Autodesk Inventor part; units mm, degrees
ref_plane "YZ Plane" through (0, 0, 0) normal (1, 0, 0) x (0, 1, 0)
ref_plane "XZ Plane" through (0, 0, 0) normal (0, 1, 0) x (-1, 0, 0)
ref_plane "XY Plane" through (0, 0, 0) normal (0, 0, 1) x (1, 0, 0)
sketch "Sketch1" plane through (0, 0, 0) normal (0, 0, 1) x (1, 0, 0)
  line L0 (-15, -10) -> (15, -10)
  line L1 (15, -10) -> (15, 10)
  line L2 (15, 10) -> (-15, 10)
  line L3 (-15, 10) -> (-15, -10)
  line L4 (-15, -10) -> (15, 10) construction
  line L5 (15, -10) -> (-15, 10) construction
  point P0 (0, 0)
  dimension "d0" = 30
  dimension "d1" = 20
extrude "Extrusion1" add sketch "Sketch1" against normal blind 5
sketch "Sketch2" plane through (0, 0, 0) normal (0, 0, 1) x (1, 0, 0)
  line L0 (-15, 0) -> (15, 0)
  line L1 (15, 0) -> (15, 15)
  line L2 (15, 15) -> (-15, 15)
  line L3 (-15, 15) -> (-15, 0)
  line L4 (-15, 0) -> (15, 15) construction
  line L5 (15, 0) -> (-15, 15) construction
  line L6 (15, 10) -> (-15, 10)
  line L7 (-15, 10) -> (-15, -10)
  point P0 (0, 0)
  point P1 (0, 7.5)
  dimension "d4" = 30
  dimension "d5" = 15
  dimension "d18" = 5
extrude "Extrusion2" add sketch "Sketch2" along normal blind 15
sketch "Sketch3" plane through (0, 0, 0) normal (0, 0, 1) x (1, 0, 0)
  circle A0 centre (10, -10) radius 2
  circle A1 centre (-10, -10) radius 2
  line L0 (-15, -10) -> (15, -10)
  line L1 (-15, 0) -> (-15, -10)
  point P0 (0, 0)
  dimension "d8" = 4
  dimension "d9" = 4
  dimension "d12" = 5
  dimension "d13" = 20
sketch "Sketch4" plane through (-15, -10, 0) normal (0, -1, 0) x (1, 0, 0)
  line L0 (0, -5) -> (30, -5)
  line L1 (30, -5) -> (30, 0)
  line L2 (30, 0) -> (0, 0)
  line L3 (0, 0) -> (0, -5)
  line L4 (0, -5) -> (30, 0) construction
  line L5 (30, -5) -> (0, 0) construction
  line L6 (0, 0) -> (30, 0)
  line L7 (30, 0) -> (30, -5)
  line L8 (0, 0) -> (0, -5)
  line L9 (30, -5) -> (0, -5)
  point P0 (15, 0)
  point P1 (15, -2.5)
extrude "Extrusion3" add sketch "Sketch4" along normal blind 5
extrude "Extrusion4" cut sketch "Sketch3" against normal blind 5
sketch "Sketch5" plane through (0, 0, -5) normal (0, 0, -1) x (-1, 0, 0)
  line L0 (-8, 0) -> (8, 0)
  line L1 (8, 0) -> (8, 15)
  line L2 (8, 15) -> (-8, 15)
  line L3 (-8, 15) -> (-8, 0)
  line L4 (-8, 0) -> (8, 15) construction
  line L5 (8, 0) -> (-8, 15) construction
  line L6 (-15, 15) -> (15, 15)
  point P0 (0, 0)
  point P1 (0, 7.5)
  dimension "d16" = 16
  dimension "d21" = 15
  dimension "d22" = 0
sketch "Sketch6" plane through (0, 0, 0) normal (0, 0, -1) x (-1, 0, 0)
  line L0 (-15, 10) -> (15, 10)
  line L1 (15, 10) -> (15, 15)
  line L2 (15, 15) -> (-15, 15)
  line L3 (-15, 15) -> (-15, 10)
  line L4 (-15, 10) -> (15, 15) construction
  line L5 (15, 10) -> (-15, 15) construction
  line L6 (-15, 15) -> (15, 15)
  line L7 (15, 10) -> (-15, 10)
  line L8 (-15, 10) -> (-15, 15)
  line L9 (15, 15) -> (15, 10)
  point P0 (0, 0)
  point P1 (0, 12.5)
extrude "Extrusion5" add sketch "Sketch6" along normal blind 5
extrude "Extrusion6" cut sketch "Sketch5" against normal through all
sketch "Sketch7" plane through (0, 0, -5) normal (0, 0, -1) x (-1, 0, 0)
  circle A0 centre (-10, 8) radius 1.5
  circle A1 centre (10, 8) radius 1.5
  line L0 (-15, 15) -> (-15, -15)
  line L1 (8, 0) -> (-8, 0)
  point P0 (0, 0)
  dimension "d25" = 3
  dimension "d26" = 3
  dimension "d27" = 20
  dimension "d28" = 5
  dimension "d33" = 8
extrude "Extrusion7" cut sketch "Sketch7" against normal through all
sketch "Sketch8" plane through (15, 15, 15) normal (0, 1, 0) x (1, 0, 0)
  line L0 (0, 20) -> (-30, 20)
  line L1 (-30, 20) -> (-30, 0)
  line L2 (-30, 0) -> (0, 0)
  line L3 (0, 0) -> (0, 20)
  line L4 (0, 20) -> (-30, 0) construction
  line L5 (-30, 20) -> (0, 0) construction
  line L6 (0, 0) -> (-7, 0)
  line L7 (0, 0) -> (0, 20)
  line L8 (-23, 20) -> (-7, 20)
  line L9 (-30, 20) -> (-30, 0)
  point P0 (-15, 15)
  point P1 (-15, 10)
extrude "Extrusion8" add sketch "Sketch8" along normal blind 3
sketch "Sketch9" plane through (0, 0, -5) normal (0, 0, -1) x (-1, 0, 0)
  line L0 (-13, 4) -> (-8, 4)
  line L1 (-8, 4) -> (-8, 12)
  line L2 (-8, 12) -> (-13, 12)
  line L3 (-13, 12) -> (-13, 4)
  line L4 (-13, 4) -> (-8, 12) construction
  line L5 (-8, 4) -> (-13, 12) construction
  line L6 (8, 4) -> (13, 4)
  line L7 (13, 4) -> (13, 12)
  line L8 (13, 12) -> (8, 12)
  line L9 (8, 12) -> (8, 4)
  line L10 (8, 4) -> (13, 12) construction
  line L11 (13, 4) -> (8, 12) construction
  line L12 (-8, 0) -> (-8, 15)
  line L13 (8, 15) -> (8, 0)
  line L14 (8, 0) -> (-8, 0)
  point P0 (0, 0)
  point P1 (-10.5, 8)
  point P2 (10.5, 8)
  dimension "d34" = 5
  dimension "d35" = 5
  dimension "d36" = 8
  dimension "d37" = 8
  dimension "d38" = 8
extrude "Extrusion9" cut sketch "Sketch9" against normal blind 10
fillet "Fillet1" radius 3 2 edges at (15, 18, 5) (-15, 18, 5)
fillet "Fillet2" radius 3 3 edges at (15, 7.5, 15) (-15, 7.5, 15) (0, 18, 15)
properties part number "IR_bracket"
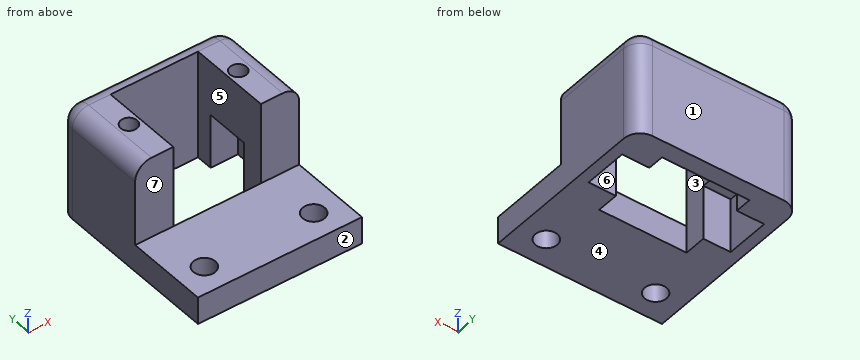
Model file for the job. Use its own axes, mm. Face numbers are marked on the shaded views. A direction names the side the tool comes from. Coordinates: 2 decimals unless noted, no trailing zeros. Write each loop counter-clockwise with the first axis right and the second up, starting at its lowest first coordinate (ties: lowest second). Pieces come first, ordered by that corner, then holes. Notation, with made-up numbers: (46.25, 52.25) - (50.25, 52.25) arc R12 cw to (50.25, 75.25) - close; hole circle Ø1 at (51.25, 54.25). An arc over 180 degrees is marked (long way). One line per item, written item: value. Start each with the question number.
1. Flat gauge pins, fed straight in: pin 1 (1.5 mm diameter, centred on x = 11, y = 7.5, fed in from -Z); pin 2 (2 mm diameter, centred on x = -12, z = 7.5, fed in from -Y); pin 3 (4.5 mm diameter, centred on x = 3.5, y = -4.5, fed in from +Z). Where does each tip first touch, or does it go through?
2. Slice it at A-A (x = 10). Write the cut outline in (y, z), plus the area to 3 significant figures.
3. Tool access for the marked faces 5, 6 and 7: list every direction of +Z, -Z, +X, -X, +Y, -Y with a clear straight run to the whole face (end or side of a thin tool).
4. Slice it at D-D (z = 11.5). Write the cut outline in (x, y), plus the area to 3 significant figures.
5. Slice it at B-B (y = 8). Write the cut outline in (x, z), plus the area to 3 significant figures.
6. Probe line 1 (Y direction, x = 10, z = -1.2); line 2 (X direction, y = -10, z = -3.9); line 3 (X direction, y = 4, z = 6.5). List the from-to ranges inside material, lowest first. Write a range as from..to.
7. Mould opens along Y. For the marked faces 1, 2, 3 and 4 say: released by +Y, released by -Y, zero draft, split by the parting line, or undercut.
Answers below:
1. pin 1: stops at z = 5
1. pin 2: stops at y = 0
1. pin 3: stops at z = 0
2. outline: (-15, -5) - (-12, -5) - (-12, 0) - (-15, 0) - close; (-8, -5) - (4, -5) - (4, 5) - (6.5, 5) - (6.5, 15) - (0, 15) - (0, 0) - (-8, 0) - close; (9.5, 5) - (12, 5) - (12, -5) - (18, -5) - (18, 12) arc R3 ccw to (15, 15) - (9.5, 15) - close
2. area: 303 mm^2
3. face 5: +Z, -Z
3. face 6: -Z
3. face 7: +Z, +X, -X, -Y
4. outline: (-15, 0) - (-8, 0) - (-8, 15) - (8, 15) - (8, 0) - (15, 0) - (15, 15) arc R3 ccw to (12, 18) - (-12, 18) arc R3 ccw to (-15, 15) - close; hole circle Ø3 at (-10, 8); hole circle Ø3 at (10, 8)
4. area: 282 mm^2
5. outline: (-15, -5) - (-13, -5) - (-13, 5) - (-11.5, 5) - (-11.5, 15) - (-12, 15) arc R3 ccw to (-15, 12) - close; (-8.5, 5) - (-8, 5) - (-8, 15) - (-8.5, 15) - close; (8, 5) - (8.5, 5) - (8.5, 15) - (8, 15) - close; (11.5, 5) - (13, 5) - (13, -5) - (15, -5) - (15, 12) arc R3 ccw to (12, 15) - (11.5, 15) - close
5. area: 116 mm^2
6. line 1: y = -15..-12, -8..4, 12..18
6. line 2: x = -15..-12, -8..8, 12..15
6. line 3: x = -15..-8, 8..15
7. face 1: released by +Y
7. face 2: released by -Y
7. face 3: undercut
7. face 4: zero draft
